Geometry: final body of the model. Coordinates: model frame, mm. Face numbers are marked on the shaded views. A direction names the side the tool comes from. Give positions to 0.01 mm unless a question says otherwise; leave off trailing zeros. Write each loop counter-clockwise with the first axis right and the second up, starting at its lowest first coordinate (ties: lowest second). Pieces come first, ordered by that corner, then holes. Notation, with made-up numbers: M 23.5,21 L 59.5,21 A11 cw 59.5,25 Z; hole C 42.25,77 d10. An arc over 180 degrees is marked long. Use a Markdown table: item, result. Add a question column.
(1) Cut plane D-D (x = -8.5). Output: boundary loops of the cut face in (y, z).
(2) Cut plane B-B (y = 6). Output: boundary loops of the cut face in (x, z).
(3) Material intervals for L1, parallel to X at y = 11.7, z = 1.15; L2, parallel to Y at x = 29.2, z = 0.65; L3, parallel to Z at x = 19.5, y = -4.5, sorted ascending.
(4) Cut plane A-A (x = -22.5). Output: boundary loops of the cut face in (y, z), plus the area to 3 significant figures.
(5) Pin query (flat end, axial travel): pin 1 Ø1.5 at (y, z) = (-13.5, 3) entering from -X; pin 2 Ø1 at (x, z) = (26, 3.5) entering from +Y; pin 3 Ø2.5 at (y, z) = (12, 6) entering from +X. Return the tip coordinate at first contact, or that it passes through.
(6) Draft query along Y for the marked faces 1, 2 and 3. Return one class per face: released by +Y, released by -Y, zero draft, split by the parting line, or undercut.
(7) Reachability of the marked faces 4, 5 and 6 from +Z, -Z, +X, -X, +Y, -Y: full face, straight path, thin tool, end or side. Return the list, or none.
(8) Cut plane C-C (z = 8.75). Output: boundary loops of the cut face in (x, y), plus the area to 3 significant figures.
```python
from build123d import *

# Parameters (mm, degrees)
SKETCH_W      = 65.4
SKETCH_H      = 30.4
PAD_DEPTH     = 1.6
FILLET_R      = 3
SKETCH001_W   = 7.5
SKETCH001_H   = 4.7
SKETCH001_W_2 = 5
SKETCH001_H_2 = 12.55
SKETCH001_W_3 = 11.2
SKETCH001_H_3 = 7.4
PAD001_DEPTH  = 3
SKETCH002_R   = 1.25
POCKET_DEPTH  = 5
SKETCH003_W   = 50
SKETCH003_H   = 5
PAD002_DEPTH  = 8.5


with BuildPart() as part:
    # Sketch → Pad (new body)
    with BuildSketch(Plane.XY):
        Rectangle(SKETCH_W, SKETCH_H)
    extrude(amount=PAD_DEPTH)

    # Fillet
    fillet_edges = [part.edges().sort_by_distance(p)[0] for p in [
        (32.7, -15.2, 0.8),
        (-32.7, -15.2, 0.8),
        (-32.7, 15.2, 0.8),
        (32.7, 15.2, 0.8),
    ]]
    fillet(fillet_edges, radius=FILLET_R)

    # Sketch001 (on Face5 of Fillet) → Pad001 (join)
    with BuildSketch(Plane.XY.offset(1.6)):
        with Locations((9.85, -12.85)):
            Rectangle(SKETCH001_W, SKETCH001_H)
        with Locations((22.35, -12.85)):
            Rectangle(SKETCH001_W, SKETCH001_H)
        with Locations((-33.2, 1.925)):
            Rectangle(SKETCH001_W_2, SKETCH001_H_2)
        with Locations((-19.8, -11.5)):
            Rectangle(SKETCH001_W_3, SKETCH001_H_3)
    extrude(amount=PAD001_DEPTH)

    # Sketch002 (on Face2 of Pad001) → Pocket (cut)
    with BuildSketch(Plane(origin=(0, 0, 0), x_dir=(1, 0, 0), z_dir=(0, 0, -1))):
        with Locations((-29.2, 11.7)):
            Circle(SKETCH002_R)
        with Locations((29.2, -11.7)):
            Circle(SKETCH002_R)
        with Locations((29.2, 11.7)):
            Circle(SKETCH002_R)
        with Locations((-29.2, -11.7)):
            Circle(SKETCH002_R)
    extrude(amount=-POCKET_DEPTH, mode=Mode.SUBTRACT)

    # Sketch003 (on Face5 of Pocket) → Pad002 (join)
    with BuildSketch(Plane.XY.offset(1.6)):
        with Locations((0, 11)):
            Rectangle(SKETCH003_W, SKETCH003_H)
    extrude(amount=PAD002_DEPTH)


solid = part.part
```
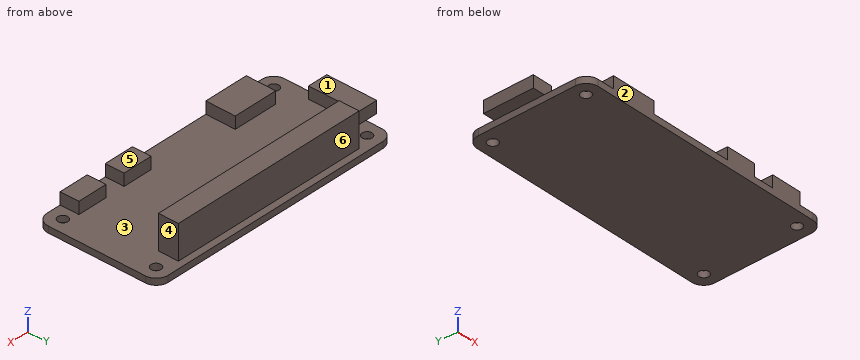
Answer list:
| question | item | result |
|---|---|---|
| 1 | outline | M -15.2,0 L 15.2,0 L 15.2,1.6 L 13.5,1.6 L 13.5,10.1 L 8.5,10.1 L 8.5,1.6 L -15.2,1.6 Z |
| 2 | outline | M -35.7,1.6 L -32.7,1.6 L -32.7,0 L 32.7,0 L 32.7,1.6 L -30.7,1.6 L -30.7,4.6 L -35.7,4.6 Z |
| 3 | L1 | -32.7 to -30.45, -27.95 to 27.95, 30.45 to 32.7 |
| 3 | L2 | -15.2 to -12.95, -10.45 to 10.45, 12.95 to 15.2 |
| 3 | L3 | 0 to 1.6 |
| 4 | outline | M -15.2,0 L 15.2,0 L 15.2,1.6 L 13.5,1.6 L 13.5,10.1 L 8.5,10.1 L 8.5,1.6 L -7.8,1.6 L -7.8,4.6 L -15.2,4.6 Z |
| 4 | area | 113 mm² |
| 5 | pin 1 | x = -25.4 |
| 5 | pin 2 | y = -10.5 |
| 5 | pin 3 | x = 25 |
| 6 | face 1 | zero draft |
| 6 | face 2 | released by -Y |
| 6 | face 3 | undercut |
| 7 | face 4 | +Z, +X, +Y |
| 7 | face 5 | +Z, +X, -X, -Y |
| 7 | face 6 | +Z, +X, -X, +Y |
| 8 | outline | M -25,8.5 L 25,8.5 L 25,13.5 L -25,13.5 Z |
| 8 | area | 250 mm² |
